Geometry check sheet. Reference: drawing and pictorial views, mm from the part's lowest x, y, z. Coordinates: 2 decimals unless noted, no trailing zeros. Write each loop counter-clockwise with the first axis right and the second up, starting at its lowest first coordinate (ties: lowest second). Pieces come first, ordered by that corner, then holes. Notation, with made-up numbers: (-32, 69) -> (-26, 69) arc R10 ccw to (-26, 82) -> close; hole circle Ø5 at (55.5, 20). An arc over 180 degrees is marked (long way). Put each result on its own line as item: value.
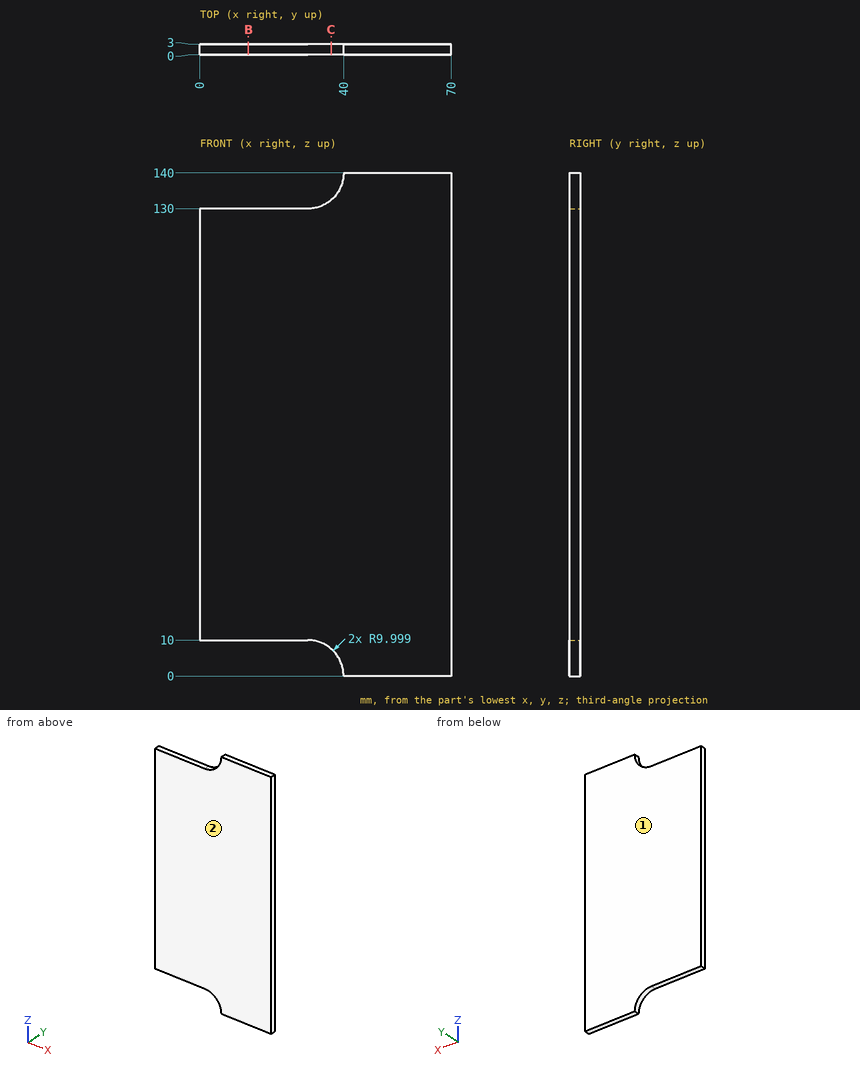
Q1. Cross-section at C-C (x = 36.5). Record the cut outline in (y, z).
Recorded:
outline: (0, 7.6) -> (3, 7.6) -> (3, 132.4) -> (0, 132.4) -> close
Q2. Material ranges on line 1 along Z through (x, y) = (5, 1.6); line 2 along Z through (x, y) = (34, 2.25) (1 decimal); line 3 along X through (y, z) = (2.7, 134), recorded low to high.
Recorded:
line 1: z = 10 to 130
line 2: z = 9.2 to 130.8
line 3: x = 38 to 70
Q3. Mould release check, pull along Y, two halves, no side actions. Record for the marked faces 1 and 2: released by +Y, released by -Y, zero draft, split by the parting line, or undercut.
Recorded:
face 1: released by +Y
face 2: released by -Y
Q4. Cross-section at B-B (x = 13.5). Record the cut outline in (y, z).
Recorded:
outline: (0, 10) -> (3, 10) -> (3, 130) -> (0, 130) -> close
